```python
from build123d import *

# Parameters (mm, degrees)
SKETCH1_R           = 5
BOSS_EXTRUDE1_DEPTH = 15
SKETCH2_R           = 7.5
BOSS_EXTRUDE2_DEPTH = 10
SKETCH3_R           = 10
BOSS_EXTRUDE3_DEPTH = 7
FILLET1_R           = 20
FILLET2_R           = 5


with BuildPart() as part:
    # Sketch1 → Boss-Extrude1 (new body)
    with BuildSketch(Plane.XY):
        Circle(SKETCH1_R)
    extrude(amount=BOSS_EXTRUDE1_DEPTH)

    # Sketch2 → Boss-Extrude2 (add)
    with BuildSketch(Plane.XY.offset(15)):
        Circle(SKETCH2_R)
    extrude(amount=BOSS_EXTRUDE2_DEPTH)

    # Sketch3 → Boss-Extrude3 (add)
    with BuildSketch(Plane.XY.offset(25)):
        Circle(SKETCH3_R)
    extrude(amount=BOSS_EXTRUDE3_DEPTH)

    # Fillet1
    # the kernel refuses this fillet: 20 mm, written as the material it adds along each edge
    with BuildSketch(Plane(origin=(0, 0, 25), x_dir=(1, 0, 0), z_dir=(0, -1, 0))) as fillet1_piece_1:
        with BuildLine():
            CenterArc((27.5, -9.682458366), FILLET1_R, 151.044975628, 28.955024372)
            Line((7.5, -9.682458366), (7.1, -9.682458366))
            Line((7.1, -9.682458366), (7.1, 0))
            Line((7.1, 0), (7.5, 0.4))
            ThreePointArc((7.5, 0.4), (8.75, 0.4), (9.65, 0.193649167))
            Line((9.65, 0.193649167), (10, 0))
        make_face()
    revolve(axis=Axis((0, 0, 25), (0, 0, 1)))

    # Fillet2
    fillet2_edges = [part.edges().sort_by_distance(p)[0] for p in [
        (-10, 0, 32),
    ]]
    fillet(fillet2_edges, radius=FILLET2_R)


solid = part.part
```
Here's how the part is built. I have some questions about the finished solid (model axes, mm). A direction names the side the tool comes from. Give positions to 0.01 mm unless a question says otherwise; leave off trailing zeros. Loops run counter-clockwise (first coordinate to the right, second up) from the corner with the lowest first, then second, coordinate; pieces in that order, holes last. Notation, with made-up numbers: M 66.5,2.5 L 121.5,2.5 A22 ccw 121.5,41.5 Z; hole C 69,53.5 d9. An arc over 180 degrees is marked long. Return JSON: item names as keys, results as strings.
Item 1: Imagine slicing it at B-B on z = 26.5. List the corners of the cut face in (x, y) for me.
A:
{"outline": "C 0,0 d20"}
Item 2: I'm going to push flat-ended pins straight in: pin 1 Ø12 at (y, z) = (-6.5, 20) entering from -X; pin 2 Ø5 at (y, z) = (-6.5, 5.5) entering from -X; pin 3 Ø4.5 at (x, y) = (-0.5, -1.5) entering from -Z; pin 4 Ø4 at (y, z) = (-2.5, 8.5) entering from -X. Where does each tip first touch, or does it pass through?
A:
{"pin 1": "stops at x = -9.48", "pin 2": "stops at x = -3", "pin 3": "stops at z = 0", "pin 4": "stops at x = -4.97"}
Item 3: Imagine slicing it at A-A on z = 10. List the corners of the cut face in (x, y) for me, then the cut area to 3 significant figures.
A:
{"outline": "C 0,0 d10", "area": "78.5 mm^2"}
Item 4: Please list where these lines run through material, in increasing order: line 1 (Y direction, x = 0.25, z = 11.5); line 2 (Y direction, x = -3.75, z = 26); line 3 (Z direction, x = 2.75, y = 5.75).
A:
{"line 1": "y = -4.99 to 4.99", "line 2": "y = -9.27 to 9.27", "line 3": "z = 15 to 31.81"}
Item 5: On a 3-axis mill with a long thin cutter (end or side, diameter ignored), from which of +Z, -Z, +X, -X, +Y, -Y can I reach the whole of each face in a straight line? I mean faces 1 (the flat face through (0, 0, 0)), 2 (the flat face through (2, -5, 15)). Say none if no direction works.
A:
{"face 1": "-Z, +X, -X, +Y, -Y", "face 2": "-Z"}
